Here's how the part is built. I have some questions about the finished solid (model axes, mm). A direction names the side the tool comes from. Round coordinates to 2 decimals unless told otherwise and drop trailing zeros. Loops run counter-clockwise (first coordinate to the right, second up) from the corner with the lowest first, then second, coordinate; pieces in that order, holes last. Notation, with made-up numbers: M 30,-18 L 88,-18 A21 ccw 88,19 Z; hole C 21,66 d6. An arc over 180 degrees is marked long. Answer as a JSON object with one key per item and string values.
from build123d import *

# Parameters (mm, degrees)
F1_DEPTH     = 8.89
F2_R         = 1.5875
F2_R_2       = 1.8513271914
F3_DEPTH     = 3.176
F5_DEPTH     = 38.101
F6_T1_DEPTH  = 17.78
F6_T6_DEPTH  = 17.78
F6_S8_R      = 6.223
F6_T9_DEPTH  = 11
F6_T13_DEPTH = 17.78
F6_S16_R     = 6.223
F6_T17_DEPTH = 11
F6_T21_DEPTH = 17.78
F6_S23_R     = 6.223
F6_T24_DEPTH = 11
F6_T28_DEPTH = 17.78
F6_S30_R     = 6.223
F6_T31_DEPTH = 11
F6_T35_DEPTH = 17.78
F6_S37_R     = 6.223
F6_T38_DEPTH = 11
F7_R         = 1.6002


# Not quite as in the source:
# - a fillet or chamfer that OpenCascade refuses, or shapes differently, is made with other operations: its cross-section is extruded or revolved along the edge and cut away or added


with BuildPart() as f1:
    # F0 (on Front) → F1 (new body, symmetric)
    with BuildSketch(Plane.XZ):
        Polygon((-38.1, 3.175), (-38.1, 0), (-22.225, 0), (-22.225, 34.925), (22.225, 34.925), (22.225, 0), (38.1, 0), (38.1, 3.175), (25.4, 3.175), (25.4, 38.1), (-25.4, 38.1), (-25.4, 3.175), align=None)
    extrude(amount=F1_DEPTH, both=True)

    # F2 (on face) → F3 (cut, through all)
    with BuildSketch(Plane.XY.offset(3.175)):
        with Locations((-31.75, 0)):
            Circle(F2_R)
        with Locations((31.75, 0)):
            Circle(F2_R_2)
    extrude(amount=-F3_DEPTH, mode=Mode.SUBTRACT)

    # F4 (on face) → F5 (cut, through all)
    with BuildSketch(Plane.XY.offset(38.1)):
        with BuildLine():
            Line((19.2827675977, 5.207), (12.4672324023, 5.207))
            ThreePointArc((12.4672324023, 5.207), (9.652, 0), (12.4672324023, -5.207))
            Line((12.4672324023, -5.207), (19.2827675977, -5.207))
            ThreePointArc((19.2827675977, -5.207), (22.098, 0), (19.2827675977, 5.207))
        make_face()
    extrude(amount=-F5_DEPTH, mode=Mode.SUBTRACT)

    # F6: fillet of radius 5.08 on 2 edges, made by hand

    # F6_s2 → F6_t1 (join)
    with BuildSketch(Plane.XZ.offset(-8.89)):
        with BuildLine():
            ThreePointArc((-22.225, 29.845), (-20.7371024484, 33.4371024484), (-17.145, 34.925))
            Line((-17.145, 34.925), (-22.225, 34.925))
            Line((-22.225, 34.925), (-22.225, 29.845))
        make_face()
    extrude(amount=F6_T1_DEPTH)


with BuildPart() as f6_tool4:
    # F6_s5 → F6_t6 (new body)
    with BuildSketch(Plane.XZ.offset(-8.89)):
        with BuildLine():
            ThreePointArc((17.145, 34.925), (20.7371024484, 33.4371024484), (22.225, 29.845))
            Line((22.225, 29.845), (22.225, 34.925))
            Line((22.225, 34.925), (17.145, 34.925))
        make_face()
    extrude(amount=F6_T6_DEPTH)

    split(bisect_by=Plane.XZ.offset(-5.207), keep=Keep.BOTTOM)

    # F6_s8 → F6_t9 (cut, symmetric)
    with BuildSketch(Plane.XY.offset(32.4)):
        with Locations((15.875, 0)):
            Circle(F6_S8_R)
    extrude(amount=F6_T9_DEPTH, both=True, mode=Mode.SUBTRACT)


with BuildPart() as f1_1:
    add(f1.part)

    # F6_t3: union F6_tool4
    add(f6_tool4.part)


with BuildPart() as f6_tool11:
    # F6_s12 → F6_t13 (new body)
    with BuildSketch(Plane.XZ.offset(-8.89)):
        with BuildLine():
            ThreePointArc((17.145, 34.925), (20.7371024484, 33.4371024484), (22.225, 29.845))
            Line((22.225, 29.845), (22.225, 34.925))
            Line((22.225, 34.925), (17.145, 34.925))
        make_face()
    extrude(amount=F6_T13_DEPTH)

    split(bisect_by=Plane.XZ.offset(5.207), keep=Keep.BOTTOM)

    split(bisect_by=Plane.XZ.offset(-5.207), keep=Keep.TOP)

    # F6_s16 → F6_t17 (cut, symmetric)
    with BuildSketch(Plane.XY.offset(32.4)):
        with Locations((15.875, 0)):
            Circle(F6_S16_R)
    extrude(amount=F6_T17_DEPTH, both=True, mode=Mode.SUBTRACT)


with BuildPart() as f1_2:
    add(f1_1.part)

    # F6_t10: union F6_tool11
    add(f6_tool11.part)


with BuildPart() as f6_tool19:
    # F6_s20 → F6_t21 (new body)
    with BuildSketch(Plane.XZ.offset(-8.89)):
        with BuildLine():
            ThreePointArc((17.145, 34.925), (20.7371024484, 33.4371024484), (22.225, 29.845))
            Line((22.225, 29.845), (22.225, 34.925))
            Line((22.225, 34.925), (17.145, 34.925))
        make_face()
    extrude(amount=F6_T21_DEPTH)

    split(bisect_by=Plane.XZ.offset(-5.207), keep=Keep.BOTTOM)

    # F6_s23 → F6_t24 (intersect, symmetric)
    with BuildSketch(Plane.XY.offset(32.4)):
        with Locations((15.875, 0)):
            Circle(F6_S23_R)
    extrude(amount=F6_T24_DEPTH, both=True, mode=Mode.INTERSECT)


with BuildPart() as f1_3:
    add(f1_2.part)

    # F6_t18: union F6_tool19
    add(f6_tool19.part)


with BuildPart() as f6_tool26:
    # F6_s27 → F6_t28 (new body)
    with BuildSketch(Plane.XZ.offset(-8.89)):
        with BuildLine():
            ThreePointArc((17.145, 34.925), (20.7371024484, 33.4371024484), (22.225, 29.845))
            Line((22.225, 29.845), (22.225, 34.925))
            Line((22.225, 34.925), (17.145, 34.925))
        make_face()
    extrude(amount=F6_T28_DEPTH)

    split(bisect_by=Plane.XZ.offset(5.207), keep=Keep.TOP)

    # F6_s30 → F6_t31 (cut, symmetric)
    with BuildSketch(Plane.XY.offset(32.4)):
        with Locations((15.875, 0)):
            Circle(F6_S30_R)
    extrude(amount=F6_T31_DEPTH, both=True, mode=Mode.SUBTRACT)


with BuildPart() as f1_4:
    add(f1_3.part)

    # F6_t25: union F6_tool26
    add(f6_tool26.part)


with BuildPart() as f6_tool33:
    # F6_s34 → F6_t35 (new body)
    with BuildSketch(Plane.XZ.offset(-8.89)):
        with BuildLine():
            ThreePointArc((17.145, 34.925), (20.7371024484, 33.4371024484), (22.225, 29.845))
            Line((22.225, 29.845), (22.225, 34.925))
            Line((22.225, 34.925), (17.145, 34.925))
        make_face()
    extrude(amount=F6_T35_DEPTH)

    split(bisect_by=Plane.XZ.offset(5.207), keep=Keep.TOP)

    # F6_s37 → F6_t38 (intersect, symmetric)
    with BuildSketch(Plane.XY.offset(32.4)):
        with Locations((15.875, 0)):
            Circle(F6_S37_R)
    extrude(amount=F6_T38_DEPTH, both=True, mode=Mode.INTERSECT)


with BuildPart() as f1_5:
    add(f1_4.part)

    # F6_t32: union F6_tool33
    add(f6_tool33.part)

    # F7
    f7_edges = [f1_5.edges().sort_by_distance(p)[0] for p in [
        (-25.4, 0, 3.175),
        (25.4, 0, 3.175),
    ]]
    fillet(f7_edges, radius=F7_R)


solid = f1_5.part
Item 1: I want a section at C-C, the plane z = 18.5. Please give me the cut outline in (x, y) (3 decimals), then the cut area to 3 significant figures.
Resolved:
{"outline": "M -25.4,-8.89 L -22.225,-8.89 L -22.225,8.89 L -25.4,8.89 Z; M 22.225,-8.89 L 25.4,-8.89 L 25.4,8.89 L 22.225,8.89 Z", "area": "113 mm²"}
Item 2: I'm going to push flat-ended pins straight in: pin 1 Ø3 at (y, z) = (-4, 29) entering from -X; pin 2 Ø9 at (x, y) = (31.5, -3) entering from +Z (3 decimals); pin 3 Ø1.5 at (y, z) = (-6.5, 34) entering from +X. Where does each tip first touch, or does it pass through?
Resolved:
{"pin 1": "x = -25.4", "pin 2": "z = 3.175", "pin 3": "x = 25.4"}
Item 3: I want a section at A-A, the plane x = -31.75. Please give me the cut outline in (y, z) (1 decimal).
Resolved:
{"outline": "M -8.9,0 L -1.6,0 L -1.6,3.2 L -8.9,3.2 Z; M 1.6,0 L 8.9,0 L 8.9,3.2 L 1.6,3.2 Z"}
Item 4: If we mould it in two halves opening along X, with no side actions, what happens to faces 5 (the face through (9.653, 0.086, 36.535)), 6 (the face through (25.4, 0, 21)), 7 (the face through (5, -8.89, 36)), 8 (the face through (-30.236, 0.477, 1.61))? For each: pulls with the +X half, pulls with the -X half, needs draft (parallel to the pull), parting line crosses it, or undercut.
Resolved:
{"face 5": "undercut", "face 6": "pulls with the +X half", "face 7": "needs draft", "face 8": "undercut"}
Item 5: Please list where these lines run through material, in increasing order: probe 1 along Y at (x, z) = (31.75, 0.75); probe 2 along X at (y, z) = (3.25, 21) (3 decimals); probe 3 along Y at (x, z) = (-31.75, 1.45). Write a range as from..to.
Resolved:
{"probe 1": "-8.89..-1.85, 1.85..8.89", "probe 2": "-25.4..-22.225, 22.225..25.4", "probe 3": "-8.89..-1.59, 1.59..8.89"}
Item 6: I want a section at D-D, the plane y = 4. Please give me the cut outline in (x, z) (3 decimals), then the cut area to 3 significant figures.
Resolved:
{"outline": "M -38.1,0 L -22.225,0 L -22.225,29.845 A5.08 cw -17.145,34.925 L 11.108,34.925 L 11.108,38.1 L -25.4,38.1 L -25.4,4.775 A1.6 cw -27,3.175 L -38.1,3.175 Z; M 20.642,33.53 A5.08 cw 22.225,29.845 L 22.225,0 L 38.1,0 L 38.1,3.175 L 27,3.175 A1.6 cw 25.4,4.775 L 25.4,38.1 L 20.642,38.1 Z", "area": "444 mm²"}
Item 7: I want a section at B-B, the plane y = 0. Please give me the cut outline in (x, z) (1 decimal).
Resolved:
{"outline": "M -38.1,0 L -33.3,0 L -33.3,3.2 L -38.1,3.2 Z; M -30.2,0 L -22.2,0 L -22.2,29.8 A5.1 cw -17.1,34.9 L 9.7,34.9 L 9.7,38.1 L -25.4,38.1 L -25.4,4.8 A1.6 cw -27,3.2 L -30.2,3.2 Z; M 22.1,31 A5.1 cw 22.2,29.8 L 22.2,0 L 29.9,0 L 29.9,3.2 L 27,3.2 A1.6 cw 25.4,4.8 L 25.4,38.1 L 22.1,38.1 Z; M 33.6,0 L 38.1,0 L 38.1,3.2 L 33.6,3.2 Z"}
Item 8: On a 3-axis mill with a long thin cutter (end or side, diameter ignored), from which of +Z, -Z, +X, -X, +Y, -Y can I reach the whole of each face in a straight line? I mean faces 1 (the face through (34, 0, 3.175)), 2 (the face through (16, 5.207, 36)), 3 (the face through (-34, 0, 3.175)), 4 (the face through (-20.776, 0.124, 33.397)). Say none if no direction works.
Resolved:
{"face 1": "+Z, +X, +Y, -Y", "face 2": "+Z, -Z", "face 3": "+Z, -X, +Y, -Y", "face 4": "-Z, +Y, -Y"}
